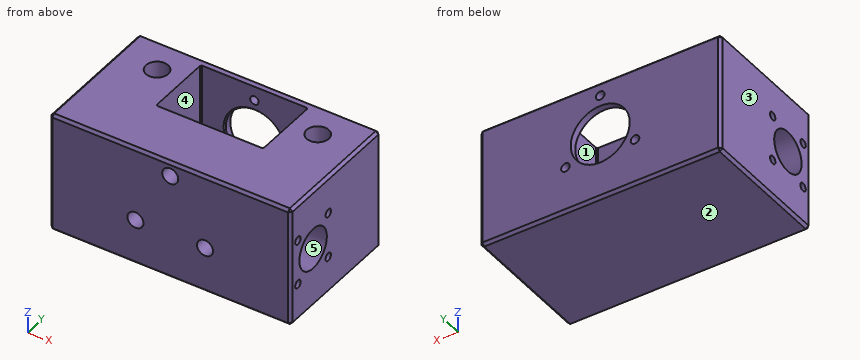
from build123d import *

# Parameters (mm, degrees)
SKETCH1_W           = 90
SKETCH1_H           = 45
BOSS_EXTRUDE1_DEPTH = 50
SKETCH2_R           = 4.15
CUT_EXTRUDE1_DEPTH  = 28.296664924
SKETCH3_R           = 7.65
CUT_EXTRUDE2_DEPTH  = 106.386194542
SKETCH4_R           = 1.5
CUT_EXTRUDE3_DEPTH  = 10
CHAMFER1_SIZE       = 1
SKETCH6_W           = 40
SKETCH6_H           = 25
CUT_EXTRUDE5_DEPTH  = 38
CUT_EXTRUDE4_REACH  = 72.931
SKETCH5_R           = 1.6
SKETCH5_R_2         = 11
CUT_EXTRUDE6_REACH  = 72.931
SKETCH8_R           = 3
CHAMFER2_SIZE       = 0.5


with BuildPart() as part:
    # Sketch1 → Boss-Extrude1 (new body)
    with BuildSketch(Plane(origin=(0, 0, 0), x_dir=(1, 0, 0), z_dir=(0, 1, 0))):
        Rectangle(SKETCH1_W, SKETCH1_H)
    extrude(amount=BOSS_EXTRUDE1_DEPTH)

    # Sketch2 → Cut-Extrude1 (cut)
    with BuildSketch(Plane.XY.offset(22.5)):
        with Locations((-30, 37.5)):
            Circle(SKETCH2_R)
        with Locations(Location((30, 37.5, 0), (0, 0, 180))):
            Circle(SKETCH2_R)
    extrude(amount=-CUT_EXTRUDE1_DEPTH, mode=Mode.SUBTRACT)

    # Sketch3 → Cut-Extrude2 (cut, through all)
    with BuildSketch(Plane(origin=(45, 0, 0), x_dir=(0, 0, -1), z_dir=(1, 0, 0))):
        with Locations((0, 12.5)):
            Circle(SKETCH3_R)
    extrude(amount=-CUT_EXTRUDE2_DEPTH, mode=Mode.SUBTRACT)

    # Sketch4 → Cut-Extrude3 (cut)
    with BuildSketch(Plane(origin=(45, 0, 0), x_dir=(0, 0, -1), z_dir=(1, 0, 0))):
        with Locations((-8.485281374, 20.985281374)):
            Circle(SKETCH4_R)
        with Locations((8.485281374, 20.985281374)):
            Circle(SKETCH4_R)
        with Locations((8.485281374, 4.014718626)):
            Circle(SKETCH4_R)
        with Locations((-8.485281374, 4.014718626)):
            Circle(SKETCH4_R)
    cut_extrude3 = extrude(amount=-CUT_EXTRUDE3_DEPTH, mode=Mode.SUBTRACT)

    # Mirror1: Cut-Extrude3 across plane
    add(cut_extrude3.mirror(Plane(origin=(0, 0, 0), x_dir=(0, 0, 1), z_dir=(1, 0, 0))), mode=Mode.SUBTRACT)

    # Chamfer1
    chamfer1_edges = [part.edges().sort_by_distance(p)[0] for p in [
        (-45, 50, 0),
        (0, 50, 22.5),
        (45, 50, 0),
        (0, 0, 22.5),
        (-45, 0, 0),
        (0, 0, -22.5),
        (45, 0, 0),
        (45, 25, 22.5),
        (-45, 25, 22.5),
        (-45, 25, -22.5),
        (45, 25, -22.5),
        (0, 50, -22.5),
    ]]
    chamfer(chamfer1_edges, length=CHAMFER1_SIZE)

    # Sketch6 → Cut-Extrude5 (cut)
    with BuildSketch(Plane.XY.offset(22.5)):
        with Locations((0, 34.5)):
            Rectangle(SKETCH6_W, SKETCH6_H)
    extrude(amount=-CUT_EXTRUDE5_DEPTH, mode=Mode.SUBTRACT)

    # Sketch5 → Cut-Extrude4 (cut, up to next)
    with BuildSketch(Plane(origin=(0, 50, 0), x_dir=(1, 0, 0), z_dir=(0, 1, 0)), mode=Mode.PRIVATE) as cut_extrude4_sk1:
        with Locations(Location((0, -17.164837936, 0), (0, 0, 270))):
            Circle(SKETCH5_R)
    cut_extrude4_tool1 = extrude(cut_extrude4_sk1.sketch, amount=-CUT_EXTRUDE4_REACH, mode=Mode.PRIVATE) & part.part
    # Sketch5 → Cut-Extrude4 (cut, up to next)
    with BuildSketch(Plane(origin=(0, 50, 0), x_dir=(1, 0, 0), z_dir=(0, 1, 0)), mode=Mode.PRIVATE) as cut_extrude4_sk2:
        with Locations(Location((-12.990381057, 5.335162064, 0), (0, 0, 270))):
            Circle(SKETCH5_R)
    cut_extrude4_tool2 = extrude(cut_extrude4_sk2.sketch, amount=-CUT_EXTRUDE4_REACH, mode=Mode.PRIVATE) & part.part
    # Sketch5 → Cut-Extrude4 (cut, up to next)
    with BuildSketch(Plane(origin=(0, 50, 0), x_dir=(1, 0, 0), z_dir=(0, 1, 0)), mode=Mode.PRIVATE) as cut_extrude4_sk3:
        with Locations(Location((12.990381057, 5.335162064, 0), (0, 0, 270))):
            Circle(SKETCH5_R)
    cut_extrude4_tool3 = extrude(cut_extrude4_sk3.sketch, amount=-CUT_EXTRUDE4_REACH, mode=Mode.PRIVATE) & part.part
    # Sketch5 → Cut-Extrude4 (cut, up to next)
    with BuildSketch(Plane(origin=(0, 50, 0), x_dir=(1, 0, 0), z_dir=(0, 1, 0)), mode=Mode.PRIVATE) as cut_extrude4_sk4:
        with Locations(Location((0, -2.164837936, 0), (0, 0, 270))):
            Circle(SKETCH5_R_2)
    cut_extrude4_tool4 = extrude(cut_extrude4_sk4.sketch, amount=-CUT_EXTRUDE4_REACH, mode=Mode.PRIVATE) & part.part
    add(cut_extrude4_tool1.solids().sort_by_distance((0, 50, 17.164838))[0], mode=Mode.SUBTRACT)
    add(cut_extrude4_tool2.solids().sort_by_distance((-12.990381, 50, -5.335162))[0], mode=Mode.SUBTRACT)
    add(cut_extrude4_tool3.solids().sort_by_distance((12.990381, 50, -5.335162))[0], mode=Mode.SUBTRACT)
    add(cut_extrude4_tool4.solids().sort_by_distance((0, 50, 2.164838))[0], mode=Mode.SUBTRACT)

    # Sketch8 → Cut-Extrude6 (cut, up to next)
    with BuildSketch(Plane.XZ, mode=Mode.PRIVATE) as cut_extrude6_sk1:
        with Locations(Location((0, 17.164837936, 0), (0, 0, 270))):
            Circle(SKETCH8_R)
    cut_extrude6_tool1 = extrude(cut_extrude6_sk1.sketch, amount=-CUT_EXTRUDE6_REACH, mode=Mode.PRIVATE) & part.part
    # Sketch8 → Cut-Extrude6 (cut, up to next)
    with BuildSketch(Plane.XZ, mode=Mode.PRIVATE) as cut_extrude6_sk2:
        with Locations(Location((12.990381057, -5.335162064, 0), (0, 0, 270))):
            Circle(SKETCH8_R)
    cut_extrude6_tool2 = extrude(cut_extrude6_sk2.sketch, amount=-CUT_EXTRUDE6_REACH, mode=Mode.PRIVATE) & part.part
    # Sketch8 → Cut-Extrude6 (cut, up to next)
    with BuildSketch(Plane.XZ, mode=Mode.PRIVATE) as cut_extrude6_sk3:
        with Locations(Location((-12.990381057, -5.335162064, 0), (0, 0, 270))):
            Circle(SKETCH8_R)
    cut_extrude6_tool3 = extrude(cut_extrude6_sk3.sketch, amount=-CUT_EXTRUDE6_REACH, mode=Mode.PRIVATE) & part.part
    add(cut_extrude6_tool1.solids().sort_by_distance((0, 0, 17.164838))[0], mode=Mode.SUBTRACT)
    add(cut_extrude6_tool2.solids().sort_by_distance((12.990381, 0, -5.335162))[0], mode=Mode.SUBTRACT)
    add(cut_extrude6_tool3.solids().sort_by_distance((-12.990381, 0, -5.335162))[0], mode=Mode.SUBTRACT)

    # Chamfer2
    chamfer2_edges = [part.edges().sort_by_distance(p)[0] for p in [
        (20, 34.5, -15.5),
        (20, 47, 3.5),
        (0, 22, -15.5),
        (20, 22, 3.5),
        (-20, 34.5, -15.5),
        (-20, 22, 3.5),
        (0, 47, -15.5),
        (-20, 47, 3.5),
        (0, 47, -8.835162064),
    ]]
    chamfer(chamfer2_edges, length=CHAMFER2_SIZE)


solid = part.part
Geometry check sheet. Reference: the model listing, model coordinates, mm. Face numbers are marked on the shaded views. A direction names the side the tool comes from. Give positions to 0.01 mm unless a question says otherwise; leave off trailing zeros. Order: outer loops, then holes, each group sorted by start corner. A loop starts at its lowest first (then second) coordinate and runs counter-clockwise, first axis right, second up.
1. Scan lines: line 1 (X direction, y = 30, z = 11.5); line 2 (Y direction, x = 30, z = 0); line 3 (Y direction, x = -11, z = 8.5). Record each from-to range of solid material in increasing order.
Completed:
line 1: x = -45 to -20, 20 to 45
line 2: y = 0 to 4.85, 20.15 to 33.35, 41.65 to 50
line 3: y = 0 to 22, 47 to 50
2. Draft check along X on the marked faces 3, 4 and 5. Enter one of: pulls with the +X half, pulls with the -X half, needs draft (parallel to the pull), parting line crosses it, or undercut.
Completed:
face 3: pulls with the -X half
face 4: undercut
face 5: needs draft
3. Sectioned sample at B-B (y = 37.5). Record the boundary of the cut face in (x, z).
Completed:
outline: (-45, -21.5) - (-44, -22.5) - (44, -22.5) - (45, -21.5) - (45, 21.5) - (44, 22.5) - (34.15, 22.5) - (34.15, -5.8) - (25.85, -5.8) - (25.85, 22.5) - (20, 22.5) - (20, -15) - (19.5, -15.5) - (-19.5, -15.5) - (-20, -15) - (-20, 22.5) - (-25.85, 22.5) - (-25.85, -5.8) - (-34.15, -5.8) - (-34.15, 22.5) - (-44, 22.5) - (-45, 21.5) - close
4. Depth check by flat-ended pin: pin 1 (2.5 mm diameter, centred on y = 20.99, z = -8.49, fed in from -X); pin 2 (1.5 mm diameter, centred on y = 4, z = 8, fed in from +X); pin 3 (5.5 mm diameter, centred on x = 12.99, z = -5.34, fed in from -Y); pin 4 (9 mm diameter, centred on y = 12.5, z = 0, fed in from -X). Enter the tip coordinate at first touch or a pass-through.
Completed:
pin 1: stops at x = -35
pin 2: stops at x = 35
pin 3: stops at y = 47
pin 4: passes through
5. Sectioned sample at A-A (x = -22). Record the boundary of the cut face in (y, z), then the cut area to 3 significant figures.
Completed:
outline: (0, -21.5) - (1, -22.5) - (49, -22.5) - (50, -21.5) - (50, 21.5) - (49, 22.5) - (1, 22.5) - (0, 21.5) - close; hole circle Ø15.3 at (12.5, 0)
area: 2,060 mm2
6. Sectioned sample at C-C (y = 12.5). Record the boundary of the cut face in (x, z), then the cut area to 3 significant figures.
Completed:
outline: (-45, -21.5) - (-44, -22.5) - (44, -22.5) - (45, -21.5) - (45, -7.65) - (14.9, -7.65) arc R3 cw to (11.08, -7.65) - (-11.08, -7.65) arc R3 cw to (-14.9, -7.65) - (-45, -7.65) - close; (-45, 7.65) - (45, 7.65) - (45, 21.5) - (44, 22.5) - (-44, 22.5) - (-45, 21.5) - close; hole circle Ø6 at (0, 17.16)
area: 2,640 mm2
7. Sectioned sample at D-D (z = 0). State how many separate pieces and enclosed holes the cut face has, then the cut area to 3 significant figures.
Completed:
separate pieces: 2
enclosed holes: 2
area: 1,950 mm2
8. Access from +Z, -Z, +X, -X, +Y, -Y to the whole of each face (thin tool, end or side, straight path). Record for the marked faces 1 and 2.
Completed:
face 1: +Z
face 2: -Z, +X, -X, +Y, -Y
